from build123d import *

# Parameters (mm, degrees)
F0_W     = 22
F0_H     = 80
F1_DEPTH = 12
F2_R     = 1.75
F3_DEPTH = 25
F4_SIZE  = 1.5
F5_R     = 4
F6_DEPTH = 4
F8_D     = 5


with BuildPart() as f1:
    # F0 (on Top) → F1 (new body)
    with BuildSketch(Plane.XY):
        Rectangle(F0_W, F0_H)
    extrude(amount=F1_DEPTH)

    # F2 (on face) → F3 (cut)
    with BuildSketch(Plane.YZ.offset(11)):
        with Locations((-16, 6)):
            Circle(F2_R)
    extrude(amount=-F3_DEPTH, mode=Mode.SUBTRACT)

    # F4
    f4_edges = [f1.edges().sort_by_distance(p)[0] for p in [
        (11, -17.75, 6),
        (-11, -17.75, 6),
    ]]
    chamfer(f4_edges, length=F4_SIZE)

    # F5 (on face) → F6 (cut)
    with BuildSketch(Plane(origin=(0, 0, 0), x_dir=(1, 0, 0), z_dir=(0, 0, -1))):
        with Locations((0, 32)):
            Circle(F5_R)
    extrude(amount=-F6_DEPTH, mode=Mode.SUBTRACT)

    # F8 (through all)
    with Locations(Plane.XY.offset(12)):
        with Locations((0, 32)):
            Hole(F8_D / 2)


solid = f1.part
Verification items for the finished model (mm, model axes). A direction names the side the tool comes from. Give positions to 0.01 mm unless a question says otherwise; leave off trailing zeros. Order: outer loops, then holes, each group sorted by start corner. A loop starts at its lowest first (then second) coordinate and runs counter-clockwise, first axis right, second up. Notation, with made-up numbers: M 14.25,7 L 59.25,7 A22 ccw 59.25,41 Z; hole C 62.5,-28 d1. An arc over 180 degrees is marked long. Use one line per item in the form item = value. Start each with the question number.
Q1. Section check D-D (y = -32). Enter the section's corners in (x, z), then the cut area to 3 significant figures.
Q2. Section check A-A (z = 6). Enter the section's corners in (x, y), then the cut area to 3 significant figures.
Q3. Mould release check, pull along X, two halves, no side actions. Record for faces 1 (the flat face through (11, -1, 6)), 2 (the cylindrical face through (0.13, -15.19, 4.45)), 3 (the cylindrical face through (-0.521, -35.966, 1.972)): +X half, -X half, draft (parallel to the pull), parting line (faces both ways), or undercut.
Q4. Scan lines: line 1 along Y through (x, z) = (0, 3.15); line 2 along Z through (x, y) = (-0.75, -16); line 3 along X through (y, z) = (-32, 0.8). Record each from-to range of solid material in increasing order. Write a range as [from, to].
Q5. Section check C-C (y = -16). Enter the section's corners in (x, z), then the cut area to 4 significant figures.
Q6. Access from +Z, -Z, +X, -X, +Y, -Y to the whole of each face (thin tool, end or side, straight path). Record for faces 4 (the flat face through (0, 1, 12)), 5 (the flat face through (0, -32, 4)).
Q7. Go/stop test with flat-tipped pins: pin 1 Ø3 at (y, z) = (-16, 6) entering from +X; pin 2 Ø2.5 at (x, y) = (-1.5, -32) entering from -Z. Record where each tip stops, or that it passes through.
Q8. Section check B-B (x = 0). Enter the section's corners in (y, z).
Evaluation:
q1.outline = M -11,0 L -4,0 L -4,4 L 4,4 L 4,0 L 11,0 L 11,12 L -11,12 Z
q1.area = 232 mm2
q2.outline = M -11,-40 L 11,-40 L 11,-19.25 L 9.5,-17.75 L -9.5,-17.75 L -11,-19.25 Z; M -11,-12.75 L -9.5,-14.25 L 9.5,-14.25 L 11,-12.75 L 11,40 L -11,40 Z; hole C 0,32 d5
q2.area = 1,660 mm2
q3.face_1 = +X half
q3.face_2 = draft
q3.face_3 = undercut
q4.line_1 = [-40, -36], [-28, 29.5], [34.5, 40]
q4.line_2 = [0, 4.25], [7.75, 12]
q4.line_3 = [-11, -4], [4, 11]
q5.outline = M -11,0 L 11,0 L 11,2.75 L 9.5,4.25 L -9.5,4.25 L -11,2.75 Z; M -11,9.25 L -9.5,7.75 L 9.5,7.75 L 11,9.25 L 11,12 L -11,12 Z
q5.area = 182.5 mm2
q6.face_4 = +Z, +X, -X, +Y, -Y
q6.face_5 = -Z
q7.pin_1 = through
q7.pin_2 = 4
q8.outline = M -40,0 L -36,0 L -36,4 L -28,4 L -28,0 L 29.5,0 L 29.5,12 L -40,12 Z; M 34.5,0 L 40,0 L 40,12 L 34.5,12 Z; hole C -16,6 d3.5
